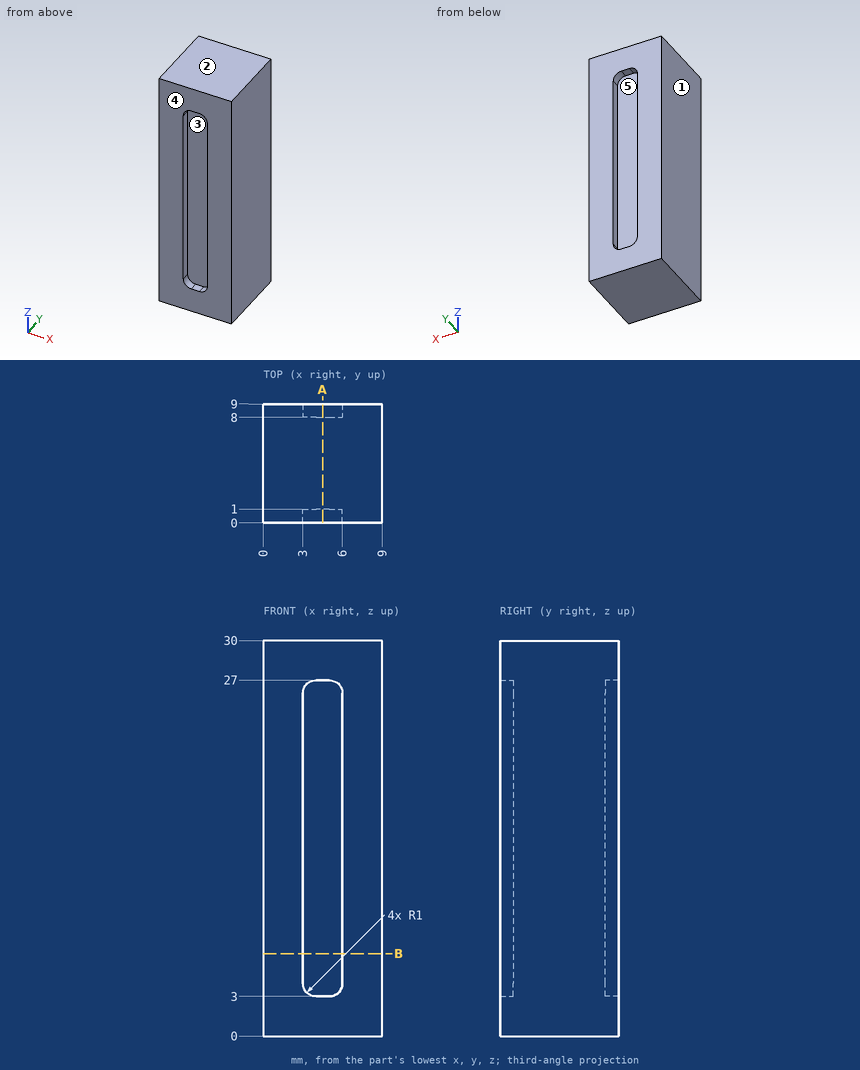
Design review of the part shown in the three views and the two pictorial views. Dimensions are in mm from the part's minimum x, y and z. A direction names the side the tool comes from. Round coordinates to 2 decimals unless told otherwise and drop trailing zeros. Order: outer loops, then holes, each group sorted by start corner. A loop starts at its lowest first (then second) coordinate and runs counter-clockwise, first axis right, second up.
Q1. We need section B-B, the plane z = 6.25. Give the boundary of the cut face in (x, y), plus the area to 3 significant figures.
Findings below:
outline: (0, 0) - (3, 0) - (3, 1) - (6, 1) - (6, 0) - (9, 0) - (9, 9) - (6, 9) - (6, 8) - (3, 8) - (3, 9) - (0, 9) - close
area: 75.0 mm2
Q2. Wall thickness on line 1 (Y direction, x = 4.5, z = 18.75); line 2 (Z direction, x = 5.5, y = 8.25): over which ranges is each line inside the solid? List them lowest first.
Findings below:
line 1: y = 1 to 8
line 2: z = 0 to 3.13, 26.87 to 30
Q3. Insertion check: P1, Ø1.5, axis at x = 2, z = 21, coming from the -Y side; P2, Ø0.9, axis at x = 4.5, z = 11, coming from the +Y side. Each pin has a flat end and moves straight along its axis. Give the tip position at first contact, or say it passes through.
Findings below:
P1: stops at y = 0
P2: stops at y = 8
Q4. Machinability: for the marked faces 4 and 5, which of the approach directions +Z, -Z, +X, -X, +Y, -Y give a long, thin tool a straight path to every point of the face, cutting with its end or side? Answer none if there is none.
Findings below:
face 4: +Z, -Z, +X, -X, -Y
face 5: +Y
Q5. Mouldability with a two-part tool opening along Z and no side actions: class the marked faces 1, 2 and 3 as pulls with the +Z half, pulls with the -Z half, needs draft (parallel to the pull), parting line crosses it, or undercut.
Findings below:
face 1: needs draft
face 2: pulls with the +Z half
face 3: undercut
Q6. We need section A-A, the plane x = 4.5. Give the boundary of the cut face in (y, z).
Findings below:
outline: (0, 0) - (9, 0) - (9, 3) - (8, 3) - (8, 27) - (9, 27) - (9, 30) - (0, 30) - (0, 27) - (1, 27) - (1, 3) - (0, 3) - close
